Design review of the part built by this model. Coordinates are the model's own, in mm. Face numbers are marked on the shaded views. Coordinates: 2 decimals unless noted, no trailing zeros. Loops run counter-clockwise (first coordinate to the right, second up) from the corner with the lowest first, then second, coordinate; pieces in that order, holes last. Notation, with made-up numbers: (50.25, 19) -> (57.25, 19) arc R15 cw to (57.25, 27) -> close; hole circle Ø6 at (64, 61.25). An arc over 180 degrees is marked (long way). Use a Markdown table: item, result. Add a question column.
Q1. Clearance check with flat-ended pins moving along their axes: pin 1 Ø3 at (x, y) = (7.5, 9.5) entering from +Z; pin 2 Ø3.5 at (x, y) = (72, 10.83) entering from +Z; pin 3 Ø0.6 at (x, y) = (21.5, 39.5) entering from +Z; pin 4 Ø8 at (x, y) = (40, 10.83) entering from -Z. State where each tip first meets the part, or that it passes through.
Q2. For probe 1 along Y at (x, z) = (8, 7.1); probe 2 along Y at (x, z) = (8, 7.6); probe 3 along Z at (x, y) = (46.5, 9.5), list the stretches that pass through material, from the lowest coordinate up.
Q3. Take a section at B-B on x = 72. Write out the cut boundary in (y, z).
Q4. Draft analysis for pull direction Y (two halves, no side actions). For the marked faces 1, 2 and 3, state which applies: pulls with the +Y half, pulls with the -Y half, needs draft (parallel to the pull), parting line crosses it, or undercut.
Q5. Take a section at A-A on x = 40. Write out the cut boundary in (y, z), plus the area to 3 significant figures.
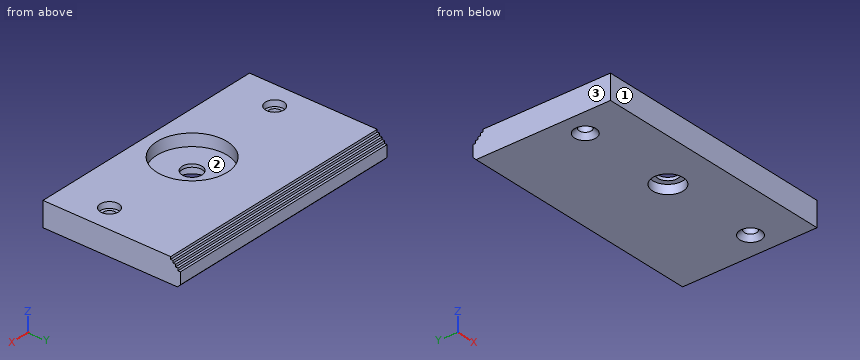
from build123d import *

# Parameters (mm, degrees)
SKETCH_1_W                     = 80
SKETCH_1_H                     = 60
EXTRUDE_1_DEPTH                = 8
HOLE_WIZARD_M3_5_1_D           = 4
HOLE_WIZARD_M3_5_1_CBORE_D     = 6
HOLE_WIZARD_M3_5_1_CBORE_DEPTH = 2
SKETCH_14_W                    = 80
SKETCH_14_H                    = 2
SKETCH_14_W_2                  = 2
SKETCH_14_H_2                  = 16
CUT_EXTRUDE_1_DEPTH            = 1
CUT_EXTRUDE_2_REACH            = 92.174
SKETCH_15_R                    = 3.25
SKETCH_17_R                    = 11.5
CUT_EXTRUDE_4_DEPTH            = 4
SKETCH_18_R                    = 5
CUT_EXTRUDE_5_DEPTH            = 3
CHAMFER_1_SIZE                 = 1.499999999
CHAMFER_1_SIZE2                = 1.500000001
CHAMFER_2_SIZE                 = 1
SKETCH_20_W                    = 80
SKETCH_20_H                    = 6
CUT_EXTRUDE_6_DEPTH            = 1
SKETCH_21_W                    = 80
SKETCH_21_H                    = 4
CUT_EXTRUDE_7_DEPTH            = 1
SKETCH_22_W                    = 80
SKETCH_22_H                    = 2
CUT_EXTRUDE_8_DEPTH            = 1
SKETCH_23_R                    = 1
CUT_EXTRUDE_9_DEPTH            = 1
CUT_EXTRUDE_10_REACH           = 92.174
SKETCH_24_W                    = 80
SKETCH_24_H                    = 15
SKETCH_25_W                    = 80
SKETCH_25_H                    = 18
EXTRUDE_2_DEPTH                = 3
CUT_EXTRUDE_11_REACH           = 92.174


with BuildPart() as part:
    # 草图1 → 凸台-拉伸1 (new body)
    with BuildSketch(Plane.XY.offset(8)):
        with Locations((40, 10.833333333)):
            Rectangle(SKETCH_1_W, SKETCH_1_H)
    extrude(amount=-EXTRUDE_1_DEPTH)

    # M3.5 六角头机械螺钉的柱形沉头孔1 (through all)
    with Locations(Plane.XY.offset(8)):
        with Locations((8, 10.833333333), (72, 10.833333333)):
            CounterBoreHole(HOLE_WIZARD_M3_5_1_D / 2, HOLE_WIZARD_M3_5_1_CBORE_D / 2, HOLE_WIZARD_M3_5_1_CBORE_DEPTH)

    # 草图14 → 切除-拉伸1 (cut)
    with BuildSketch(Plane.XY.offset(8)):
        with Locations((40, 37.833333333)):
            Rectangle(SKETCH_14_W, SKETCH_14_H)
        Polygon((15, 40.833333333), (31, 24.833333333), (32.414213562, 26.247546896), (16.414213562, 42.247546896), align=None)
        with Locations((7, 32.833333333)):
            Rectangle(SKETCH_14_W_2, SKETCH_14_H_2)
        with Locations((40, 32.833333333)):
            Rectangle(SKETCH_14_W_2, SKETCH_14_H_2)
        with Locations((73, 32.833333333)):
            Rectangle(SKETCH_14_W_2, SKETCH_14_H_2)
        Polygon((47.585786438, 26.247546896), (63.585786438, 42.247546896), (65, 40.833333333), (49, 24.833333333), align=None)
    extrude(amount=-CUT_EXTRUDE_1_DEPTH, mode=Mode.SUBTRACT)

    # 草图15 → 切除-拉伸2 (cut, up to next)
    with BuildSketch(Plane.XY.offset(8), mode=Mode.PRIVATE) as cut_extrude_2_sk1:
        with Locations((40, 10.833333333)):
            Circle(SKETCH_15_R)
    cut_extrude_2_tool1 = extrude(cut_extrude_2_sk1.sketch, amount=-CUT_EXTRUDE_2_REACH, mode=Mode.PRIVATE) & part.part
    add(cut_extrude_2_tool1.solids().sort_by_distance((40, 10.833333, 8))[0], mode=Mode.SUBTRACT)

    # 草图17 → 切除-拉伸4 (cut)
    with BuildSketch(Plane.XY.offset(8)):
        with Locations((40, 10.833333333)):
            Circle(SKETCH_17_R)
    extrude(amount=-CUT_EXTRUDE_4_DEPTH, mode=Mode.SUBTRACT)

    # 草图18 → 切除-拉伸5 (cut)
    with BuildSketch(Plane(origin=(0, 0, 0), x_dir=(-1, 0, 0), z_dir=(0, 0, -1))):
        with Locations((-40, 10.833333333)):
            Circle(SKETCH_18_R)
    extrude(amount=-CUT_EXTRUDE_5_DEPTH, mode=Mode.SUBTRACT)

    # 倒角1
    chamfer_1_edges = [part.edges().sort_by_distance(p)[0] for p in [
        (74, 10.833333333, 0),
        (10, 10.833333333, 0),
    ]]
    chamfer_1_side = [part.faces().sort_by_distance(p)[0] for p in [
        (79, 10.833333333, 0),
    ]]
    chamfer(chamfer_1_edges, length=CHAMFER_1_SIZE, length2=CHAMFER_1_SIZE2, reference=chamfer_1_side[0])

    # 倒角2
    chamfer_2_edges = [part.edges().sort_by_distance(p)[0] for p in [
        (40, 40.833333333, 0),
    ]]
    chamfer(chamfer_2_edges, length=CHAMFER_2_SIZE)

    # 草图20 → 切除-拉伸6 (cut)
    with BuildSketch(Plane.XY.offset(8)):
        with Locations((40, -16.166666667)):
            Rectangle(SKETCH_20_W, SKETCH_20_H)
    extrude(amount=-CUT_EXTRUDE_6_DEPTH, mode=Mode.SUBTRACT)

    # 草图21 → 切除-拉伸7 (cut)
    with BuildSketch(Plane.XY.offset(7)):
        with Locations((40, -17.166666667)):
            Rectangle(SKETCH_21_W, SKETCH_21_H)
    extrude(amount=-CUT_EXTRUDE_7_DEPTH, mode=Mode.SUBTRACT)

    # 草图22 → 切除-拉伸8 (cut)
    with BuildSketch(Plane.XY.offset(6)):
        with Locations((40, -18.166666667)):
            Rectangle(SKETCH_22_W, SKETCH_22_H)
    extrude(amount=-CUT_EXTRUDE_8_DEPTH, mode=Mode.SUBTRACT)

    # 草图23 → 切除-拉伸9 (cut)
    with BuildSketch(Plane.XY.offset(8)):
        with Locations((7, 24.833333333)):
            Circle(SKETCH_23_R)
        with Locations((31.707106781, 25.540440115)):
            Circle(SKETCH_23_R)
        with Locations((40, 24.833333333)):
            Circle(SKETCH_23_R)
        with Locations((48.292893219, 25.540440115)):
            Circle(SKETCH_23_R)
        with Locations((73, 24.833333333)):
            Circle(SKETCH_23_R)
    extrude(amount=-CUT_EXTRUDE_9_DEPTH, mode=Mode.SUBTRACT)

    # 草图24 → 切除-拉伸10 (cut, up to next)
    with BuildSketch(Plane.XY.offset(8), mode=Mode.PRIVATE) as cut_extrude_10_sk1:
        with Locations((40, -11.666666667)):
            Rectangle(SKETCH_24_W, SKETCH_24_H)
    cut_extrude_10_tool1 = extrude(cut_extrude_10_sk1.sketch, amount=-CUT_EXTRUDE_10_REACH, mode=Mode.PRIVATE) & part.part
    add(cut_extrude_10_tool1.solids().sort_by_distance((40, -11.666667, 8))[0], mode=Mode.SUBTRACT)

    # 草图25 → 凸台-拉伸2 (add)
    with BuildSketch(Plane.XY.offset(8)):
        with Locations((40, 31.833333333)):
            Rectangle(SKETCH_25_W, SKETCH_25_H)
    extrude(amount=-EXTRUDE_2_DEPTH)

    # 草图26 → 切除-拉伸11 (cut, up to next)
    with BuildSketch(Plane.ZY, mode=Mode.PRIVATE) as cut_extrude_11_sk1:
        Polygon((4.8, 40.833333333), (4.8, 40.033333333), (5.6, 40.033333333), (5.6, 39.233333333), (6.4, 39.233333333), (6.4, 38.433333333), (7.2, 38.433333333), (7.2, 37.633333333), (8, 37.633333333), (8, 40.833333333), align=None)
    cut_extrude_11_tool1 = extrude(cut_extrude_11_sk1.sketch, amount=-CUT_EXTRUDE_11_REACH, mode=Mode.PRIVATE) & part.part
    add(cut_extrude_11_tool1.solids().sort_by_distance((0, 39.633333, 6.8))[0], mode=Mode.SUBTRACT)


solid = part.part
Answer list:
| question | item | result |
|---|---|---|
| 1 | pin 1 | z = 6 |
| 1 | pin 2 | through |
| 1 | pin 3 | z = 6.4 |
| 1 | pin 4 | z = 3 |
| 2 | probe 1 | -4.17 to 7.83, 13.83 to 38.43 |
| 2 | probe 2 | -4.17 to 7.83, 13.83 to 37.63 |
| 2 | probe 3 | 0 to 4 |
| 3 | outline | (-4.17, 0) -> (7.33, 0) -> (8.83, 1.5) -> (8.83, 6) -> (7.83, 6) -> (7.83, 8) -> (-4.17, 8) -> close; (12.83, 1.5) -> (14.33, 0) -> (39.83, 0) -> (40.83, 1) -> (40.83, 4.8) -> (40.03, 4.8) -> (40.03, 5.6) -> (39.23, 5.6) -> (39.23, 6.4) -> (38.43, 6.4) -> (38.43, 7.2) -> (37.63, 7.2) -> (37.63, 8) -> (13.83, 8) -> (13.83, 6) -> (12.83, 6) -> close |
| 4 | face 1 | pulls with the -Y half |
| 4 | face 2 | undercut |
| 4 | face 3 | needs draft |
| 5 | outline | (-4.17, 0) -> (5.83, 0) -> (5.83, 3) -> (7.58, 3) -> (7.58, 4) -> (-0.67, 4) -> (-0.67, 8) -> (-4.17, 8) -> close; (14.08, 3) -> (15.83, 3) -> (15.83, 0) -> (39.83, 0) -> (40.83, 1) -> (40.83, 4.8) -> (40.03, 4.8) -> (40.03, 5.6) -> (39.23, 5.6) -> (39.23, 6.4) -> (38.43, 6.4) -> (38.43, 7.2) -> (37.63, 7.2) -> (37.63, 8) -> (22.33, 8) -> (22.33, 4) -> (14.08, 4) -> close |
| 5 | area | 225 mm² |
